Could you check a few things on this model? Use its own coordinates, in mm. A direction names the side the tool comes from. Give positions to 0.01 mm unless a question says otherwise; leave off trailing zeros. Order: outer loops, then holes, each group sorted by start corner. A loop starts at its lowest first (then second) coordinate and runs counter-clockwise, first axis right, second up. Notation, with made-up numbers: M 77,3 L 111,3 A24 ccw 111,20 Z; hole C 58.5,28 d6. An arc over 180 degrees is marked long. Answer in a Markdown table with one row per item. Add a question column.
```python
from build123d import *

# Parameters (mm, degrees)
SALIENTE_EXTRUIR2_DEPTH = 6
CROQUIS2_W              = 6
CROQUIS2_H              = 1
SALIENTE_EXTRUIR3_DEPTH = 6
CROQUIS3_R              = 2
CORTAR_EXTRUIR1_DEPTH   = 5.2
REDONDEO1_R             = 0.5


with BuildPart() as part:
    # Croquis1 → Saliente-Extruir2 (new body)
    with BuildSketch(Plane.XY):
        Polygon((0, 0), (-4.5, 0), (-4.5, -1.5), (-3.5, -3.2), (0, -3.2), align=None)
        Polygon((4.5, 0), (0, 0), (0, -3.2), (3.5, -3.2), (4.5, -1.5), align=None)
    extrude(amount=SALIENTE_EXTRUIR2_DEPTH)

    # Croquis2 → Saliente-Extruir3 (add)
    with BuildSketch(Plane.XY.offset(6)):
        with Locations((0, 0.5)):
            Rectangle(CROQUIS2_W, CROQUIS2_H)
    extrude(amount=-SALIENTE_EXTRUIR3_DEPTH)

    # Croquis3 → Cortar-Extruir1 (cut, through all)
    with BuildSketch(Plane(origin=(0, 1, 0), x_dir=(1, 0, 0), z_dir=(0, 1, 0))):
        with Locations((0, -3)):
            Circle(CROQUIS3_R)
    extrude(amount=-CORTAR_EXTRUIR1_DEPTH, mode=Mode.SUBTRACT)

    # Redondeo1
    redondeo1_edges = [part.edges().sort_by_distance(p)[0] for p in [
        (0, -3.2, 6),
        (-4.5, 0, 3),
        (4.5, 0, 3),
        (4.5, -1.5, 3),
        (-4.5, -1.5, 3),
        (4, -2.35, 6),
        (4.5, -0.75, 6),
        (3.75, 0, 0),
        (3.75, 0, 6),
        (-3, 0.5, 0),
        (0, 1, 6),
        (3, 0.5, 6),
        (0, 1, 0),
        (3, 0.5, 0),
        (-3.75, 0, 6),
        (-3, 0.5, 6),
        (-4.5, -0.75, 6),
        (-3.75, 0, 0),
        (4.5, -0.75, 0),
        (-4, -2.35, 6),
        (4, -2.35, 0),
        (0, -3.2, 0),
        (-4, -2.35, 0),
        (-4.5, -0.75, 0),
    ]]
    fillet(redondeo1_edges, radius=REDONDEO1_R)


solid = part.part
```
1. Suppose I cut it at A-A on z = 3. List the corners of the cut face in (x, y) for me.
2. Suppose I cut it at B-B on x = 0. List the corners of the cut face in (y, z) for me, plus the area to 3 significant figures.
3. For faces 1 (the flat face through (-3, 0.5, 3)), 2 (the cylindrical face through (3.8, -2.3, 0.1)), 3 (the flat face through (3.5, 0, 3)), which set-ups out of +Z, -Z, +X, -X, +Y, -Y let a thin tool reach every point of the face, with its end or its side?
4. Suppose I cut it at D-D on y = 0.15. List the corners of the cut face in (x, z) for me.
5. If I drill on line 1 along X through (y, z) = (-0.8, 3); line 2 along X through (y, z) = (-2.35, 3); line 3 along Z through (x, y) = (0, -1.6), over which ranges is the centre line in solid material (lowest first)? Write a range as [from, to].
6. Suppose I cut it at C-C on y = -0.9. List the corners of the cut face in (x, z) for me.
7. Will these pins go through, and if not, where does the flat tip stop? P1, Ø1, axis at y = 0, z = 2, coming from the +X side; P2, Ø0.5, axis at x = 3.5, z = 2.5, coming from the +Y side; P3, Ø0.5, axis at y = 0.5, z = 2, coming from the -X side; P4, Ø0.8, axis at y = 0.5, z = 3.5, coming from the +X side.
Findings below:
| question | item | result |
|---|---|---|
| 1 | outline | M -4.5,-1.36 A0.5 ccw -4.43,-1.62 L -3.5,-3.2 L -2,-3.2 L -2,1 L -3,1 L -3,0 L -4,0 A0.5 ccw -4.5,-0.5 Z; M 2,-3.2 L 3.5,-3.2 L 4.43,-1.62 A0.5 ccw 4.5,-1.36 L 4.5,-0.5 A0.5 ccw 4,0 L 3,0 L 3,1 L 2,1 Z |
| 2 | outline | M -3.2,0.5 A0.5 ccw -2.7,0 L 0.5,0 A0.5 ccw 1,0.5 L 1,1 L -3.2,1 Z; M -3.2,5 L 1,5 L 1,5.5 A0.5 ccw 0.5,6 L -2.7,6 A0.5 ccw -3.2,5.5 Z |
| 2 | area | 8.19 mm2 |
| 3 | face 1 | +Z, -Z, -X, +Y |
| 3 | face 2 | -Z, +X, -Y |
| 3 | face 3 | +Z, -Z, +X, +Y |
| 4 | outline | M -3,0.5 A0.5 ccw -2.5,0 L 2.5,0 A0.5 ccw 3,0.5 L 3,5.5 A0.5 ccw 2.5,6 L -2.5,6 A0.5 ccw -3,5.5 Z; hole C 0,3 d4 |
| 5 | line 1 | [-4.5, -2], [2, 4.5] |
| 5 | line 2 | [-4, -2], [2, 4] |
| 5 | line 3 | [0, 1], [5, 6] |
| 6 | outline | M -4.5,0.5 A0.5 ccw -4,0 L 4,0 A0.5 ccw 4.5,0.5 L 4.5,5.5 A0.5 ccw 4,6 L -4,6 A0.5 ccw -4.5,5.5 Z; hole C 0,3 d4 |
| 7 | P1 | x = 4.5 |
| 7 | P2 | y = 0 |
| 7 | P3 | x = -3 |
| 7 | P4 | x = 3 |
